```python
from build123d import *

# Parameters (mm, degrees)
SKETCH1_W           = 42.3
SKETCH1_H           = 42.3
SKETCH1_R           = 1.5
BOSS_EXTRUDE1_DEPTH = 48
SKETCH2_R           = 11
BOSS_EXTRUDE2_DEPTH = 2
SKETCH3_R           = 2.5
BOSS_EXTRUDE3_DEPTH = 24
FILLET1_R           = 0.5
FILLET2_R           = 0.2


with BuildPart() as part:
    # Sketch1 → Boss-Extrude1 (new body)
    with BuildSketch(Plane(origin=(0, 0, 0), x_dir=(1, 0, 0), z_dir=(0, 1, 0))):
        Rectangle(SKETCH1_W, SKETCH1_H)
        with Locations(Location((15.5, 15.5, 0), (0, 0, 270))):
            Circle(SKETCH1_R, mode=Mode.SUBTRACT)
        with Locations(Location((-15.5, 15.5, 0), (0, 0, 270))):
            Circle(SKETCH1_R, mode=Mode.SUBTRACT)
        with Locations(Location((-15.5, -15.5, 0), (0, 0, 270))):
            Circle(SKETCH1_R, mode=Mode.SUBTRACT)
        with Locations(Location((15.5, -15.5, 0), (0, 0, 270))):
            Circle(SKETCH1_R, mode=Mode.SUBTRACT)
    extrude(amount=-BOSS_EXTRUDE1_DEPTH)

    # Sketch2 → Boss-Extrude2 (add)
    with BuildSketch(Plane(origin=(0, 0, 0), x_dir=(1, 0, 0), z_dir=(0, 1, 0))):
        with Locations(Location((0, 0, 0), (0, 0, 270))):
            Circle(SKETCH2_R)
    extrude(amount=BOSS_EXTRUDE2_DEPTH)

    # Sketch3 → Boss-Extrude3 (add)
    with BuildSketch(Plane(origin=(0, 0, 0), x_dir=(1, 0, 0), z_dir=(0, 1, 0))):
        with Locations(Location((0, 0, 0), (0, 0, 270))):
            Circle(SKETCH3_R)
    extrude(amount=BOSS_EXTRUDE3_DEPTH)

    # Fillet1
    fillet1_edges = [part.edges().sort_by_distance(p)[0] for p in [
        (0, 0, -11),
    ]]
    fillet(fillet1_edges, radius=FILLET1_R)

    # Fillet2
    fillet2_edges = [part.edges().sort_by_distance(p)[0] for p in [
        (0, 2, -11),
    ]]
    fillet(fillet2_edges, radius=FILLET2_R)


solid = part.part
```
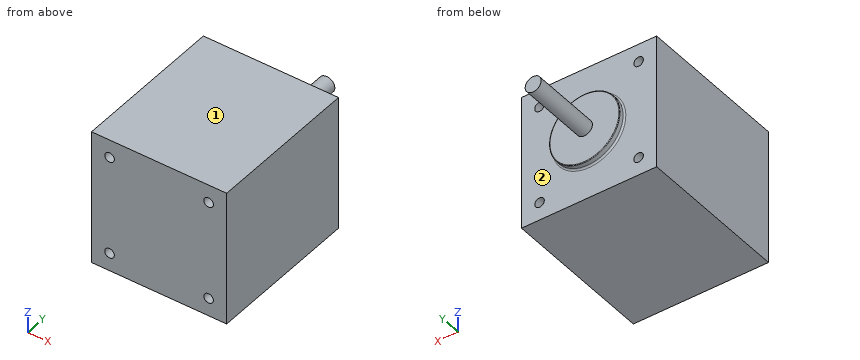
Check sheet for the modelled part. Datum: model origin and axes. Units: mm. Face numbers are marked on the shaded views. A direction names the side the tool comes from. Give positions to 0.01 mm unless a question says otherwise; leave off trailing zeros. Write each loop counter-clockwise with the first axis right and the second up, starting at its lowest first coordinate (ties: lowest second). Pieces come first, ordered by that corner, then holes.
Item 1: Cross-section at D-D (x = 0). Enter the section's corners in (y, z), and give its area (3 significant figures).
Item 2: Access from +Z, -Z, +X, -X, +Y, -Y to the whole of each face (thin tool, end or side, straight path). Record for the marked faces 1 and 2.
Item 3: Scan lines: L1, parallel to X at y = -37, z = -15.5; L2, parallel to Z at x = 15, y = -24; L3, parallel to Y at x = -17, z = -3.5. Record each from-to range of solid material in increasing order.
Item 4: Cross-section at A-A (y = -6.5). Enter the section's corners in (x, z).
Item 5: Gauge pin test, flat ends, axial feed: pin 1 (12 mm diameter, centred on x = 2.5, z = -4, fed in from +Y); pin 2 (5 mm diameter, centred on x = -15.5, z = -15.5, fed in from +Y). Record the tip position at first contact, or that the pin passes through.
Item 6: Cross-section at C-C (x = -15.5). Enter the section's corners in (y, z), and give its area (3 significant figures).
Item 7: Cross-section at B-B (z = 15.5). Enter the section's corners in (x, y).
Report:
1. outline: (-48, -21.15) - (0, -21.15) - (0, -11.5) arc R0.5 cw to (0.5, -11) - (1.8, -11) arc R0.2 ccw to (2, -10.8) - (2, -2.5) - (24, -2.5) - (24, 2.5) - (2, 2.5) - (2, 10.8) arc R0.2 ccw to (1.8, 11) - (0.5, 11) arc R0.5 cw to (0, 11.5) - (0, 21.15) - (-48, 21.15) - close
1. area: 2,180 mm2
2. face 1: +Z, +X, -X, +Y, -Y
2. face 2: +Y
3. L1: x = -21.15 to -17, -14 to 14, 17 to 21.15
3. L2: z = -21.15 to -16.91, -14.09 to 14.09, 16.91 to 21.15
3. L3: y = -48 to 0
4. outline: (-21.15, -21.15) - (21.15, -21.15) - (21.15, 21.15) - (-21.15, 21.15) - close; hole circle Ø3 at (-15.5, -15.5); hole circle Ø3 at (-15.5, 15.5); hole circle Ø3 at (15.5, -15.5); hole circle Ø3 at (15.5, 15.5)
5. pin 1: stops at y = 24
5. pin 2: stops at y = 0
6. outline: (-48, -21.15) - (0, -21.15) - (0, -17) - (-48, -17) - close; (-48, -14) - (0, -14) - (0, 14) - (-48, 14) - close; (-48, 17) - (0, 17) - (0, 21.15) - (-48, 21.15) - close
6. area: 1,740 mm2
7. outline: (-21.15, -48) - (-17, -48) - (-17, 0) - (-21.15, 0) - close; (-14, -48) - (14, -48) - (14, 0) - (-14, 0) - close; (17, -48) - (21.15, -48) - (21.15, 0) - (17, 0) - close
